```python
from build123d import *

# Parameters (mm, degrees)
SKETCH1_W           = 20
SKETCH1_H           = 110
BOSS_EXTRUDE1_DEPTH = 20
BOSS_EXTRUDE3_DEPTH = 20
BOSS_EXTRUDE4_DEPTH = 20


with BuildPart() as part:
    # Sketch1 → Boss-Extrude1 (new body)
    with BuildSketch(Plane(origin=(0, 0, 0), x_dir=(1, 0, 0), z_dir=(0, 1, 0))):
        with Locations((10, 55)):
            Rectangle(SKETCH1_W, SKETCH1_H)
    extrude(amount=BOSS_EXTRUDE1_DEPTH)

    # Sketch3 → Boss-Extrude3 (add)
    with BuildSketch(Plane(origin=(0, 0, 0), x_dir=(0, 0, -1), z_dir=(1, 0, 0))):
        Polygon((0, 7), (0, 13), (-2, 13), (-2, 14.9), (-6, 13), (-6, 7), (-2, 5.1), (-2, 7), align=None)
    extrude(amount=BOSS_EXTRUDE3_DEPTH)

    # Sketch5 → Boss-Extrude4 (add)
    with BuildSketch(Plane(origin=(0, 20, 0), x_dir=(1, 0, 0), z_dir=(0, 1, 0))):
        Polygon((13, 110), (7, 110), (7, 112), (5.1, 112), (7, 116), (13, 116), (14.9, 112), (13, 112), align=None)
    extrude(amount=-BOSS_EXTRUDE4_DEPTH)


solid = part.part
```
Check sheet for the modelled part. Datum: model origin and axes. Units: mm. A direction names the side the tool comes from. Give positions to 0.01 mm unless a question says otherwise; leave off trailing zeros. Write each loop counter-clockwise with the first axis right and the second up, starting at its lowest first coordinate (ties: lowest second). Pieces come first, ordered by that corner, then holes. Notation, with made-up numbers: (-15.75, -32) - (-7.75, -32) arc R31 ccw to (-7.75, 7) - close; hole circle Ø7 at (-25, 30.5). An arc over 180 degrees is marked (long way). Answer as a JSON object with one key per item and string values. Group by question number.
1) Thickness scan on probe 1 along Z at (x, y) = (6.75, 3.75); probe 2 along Z at (x, y) = (18.5, 7.5); probe 3 along Z at (x, y) = (10.5, 16.5). Record the ranges inside material, lowest first. Write a range as from..to.
2) Access from +Z, -Z, +X, -X, +Y, -Y to the whole of each face (thin tool, end or side, straight path). Record for faces 5 (the face through (10, 6, 2)), 6 (the face through (14, 10, -112)), 7 (the face through (10, 14, 2)), 8 (the face through (10, 20, -59)).
3) Sectioned sample at B-B (x = 11.75). Record the cut outline in (y, z).
4) Release check for a two-part mould opening along Z. For faces 1 (the face through (9.86, 13.963, 3.972)), 2 (the face through (13, 10, -111)), 3 (the face through (10, 0, -59)), 4 (the face through (10, 16, 0)) record: pulls with the +Z half, pulls with the -Z half, needs draft (parallel to the pull), parting line crosses it, or undercut.
5) Sectioned sample at A-A (y = 17.25). Record the cut outline in (x, z), then the cut area to 3 significant figures.
6) Depth check by flat-ended pin: P1, Ø1, axis at y = 6, z = -111, coming from the -X side; P2, Ø3.5, axis at x = 4, y = 13, coming from the -Z side; P3, Ø3.5, axis at x = 7.5, y = 15.5, coming from the +Z side. Enter the tip coordinate at first touch or a pass-through.
Geometry results:
{
 "1": {"probe 1": "z = -115.47..-112, -110..0", "probe 2": "z = -110..6", "probe 3": "z = -116..0"},
 "2": {"face 5": "+X, -X, -Y", "face 6": "+X, +Y, -Y", "face 7": "+X, -X, +Y", "face 8": "+Z, -Z, +X, -X, +Y"},
 "3": {"outline": "(0, -116) - (20, -116) - (20, 0) - (13, 0) - (13, 2) - (14.9, 2) - (13, 6) - (7, 6) - (5.1, 2) - (7, 2) - (7, 0) - (0, 0) - close"},
 "4": {"face 1": "pulls with the +Z half", "face 2": "undercut", "face 3": "needs draft", "face 4": "undercut"},
 "5": {"outline": "(0, -110) - (7, -110) - (7, -112) - (5.1, -112) - (7, -116) - (13, -116) - (14.9, -112) - (13, -112) - (13, -110) - (20, -110) - (20, 0) - (0, 0) - close", "area": "2,240 mm^2"},
 "6": {"P1": "stops at x = 7", "P2": "stops at z = -113.37", "P3": "stops at z = 4.42"}
}
